from build123d import *

# Parameters (mm, degrees)
F0_R     = 19.05
F1_DEPTH = 3.175
F2_R     = 17.5006
F3_DEPTH = 69.85
F4_R     = 17.5006
F5_DEPTH = 69.85
F6_R     = 9.525
F7_DEPTH = 142.876
F8_SIZE  = 1.5875


with BuildPart() as f1:
    # F0 (on Front) → F1 (new body)
    with BuildSketch(Plane.XZ):
        Circle(F0_R)
    extrude(amount=F1_DEPTH)

    # F2 (on face) → F3 (join)
    with BuildSketch(Plane.XZ.offset(3.175)):
        Circle(F2_R)
    extrude(amount=F3_DEPTH)

    # F4 (on face) → F5 (join)
    with BuildSketch(Plane(origin=(0, 0, 0), x_dir=(-1, 0, 0), z_dir=(0, 1, 0))):
        Circle(F4_R)
    extrude(amount=F5_DEPTH)

    # F6 (on face) → F7 (cut, through all)
    with BuildSketch(Plane(origin=(0, 69.85, 0), x_dir=(-1, 0, 0), z_dir=(0, 1, 0))):
        Circle(F6_R)
    extrude(amount=-F7_DEPTH, mode=Mode.SUBTRACT)

    # F8
    f8_edges = [f1.edges().sort_by_distance(p)[0] for p in [
        (-17.5006, -73.025, 0),
        (9.525, -73.025, 0),
        (9.525, 69.85, 0),
        (17.5006, 69.85, 0),
    ]]
    chamfer(f8_edges, length=F8_SIZE)


solid = f1.part
Input: part model. Units: mm. Frame: model coordinates. A direction names the side the tool comes from. Coordinates: 2 decimals unless noted, no trailing zeros. Order: outer loops, then holes, each group sorted by start corner. A loop starts at its lowest first (then second) coordinate and runs counter-clockwise, first axis right, second up.
1. Draft query along Z for faces 1 (the conical face through (15.3, -72.9, 4.8)), 2 (the cylindrical face through (7.559, -0.61, -5.796)), 3 (the flat face through (17, 0, -6)). Return one class per face: +Z half, -Z half, draft (parallel to the pull), parting line (faces both ways), or undercut.
Checked values:
face 1: parting line
face 2: undercut
face 3: draft
2. Cut plane C-C, the plane y = -49. Return loops of the section in (x, z) (3 decimals).
Checked values:
outline: circle Ø35.001 at (0, 0); hole circle Ø19.05 at (0, 0)
3. Ray query, line 1 along Z through (x, y) = (0, 11.5) (3 decimals); line 2 along Z through (x, y) = (6, 31.5); line 3 along X through (y, z) = (34, 3.5). Return the intervals inside material, ascending.
Checked values:
line 1: z = -17.501 to -9.525, 9.525 to 17.501
line 2: z = -16.44 to -7.4, 7.4 to 16.44
line 3: x = -17.15 to -8.86, 8.86 to 17.15
4. Access query for faces 4 (the cylindrical face through (-16.69, 33.65, 5.26)), 5 (the cylindrical face through (16.69, -36.83, 5.26)), 6 (the flat face through (3, -73.025, 11)). Directions: +Z, -Z, +X, -X, +Y, -Y. A direction counts if a zero-diameter tool reaches every point of the face in a straight line with its end or side. Return the directions, or none.
Checked values:
face 4: +Y
face 5: -Y
face 6: +Z, -Z, +X, -X, -Y
5. Contact query for flat-ended pins moving along their axis: P1, Ø5, axis at y = 2, z = -3.5, coming from the -X side; P2, Ø1.5, axis at x = 11.5, z = -12.5, coming from the +Y side; P3, Ø4, axis at y = -11.5, z = -1.5, coming from the -X side. Output: stop coordinate, or through.
Checked values:
P1: stops at x = -18.94
P2: stops at y = 69.53
P3: stops at x = -17.5
